Build history of the part. All positions in model axes, mm. Face numbers are marked on the shaded views. A direction names the side the tool comes from. Round coordinates to 2 decimals unless told otherwise and drop trailing zeros. Order: outer loops, then holes, each group sorted by start corner. A loop starts at its lowest first (then second) coordinate and runs counter-clockwise, first axis right, second up. Notation, with made-up numbers: M -27.75,34.5 L 18.25,34.5 A20 ccw 18.25,40.5 Z; hole C 80.5,-14.75 d1. An arc over 180 degrees is marked long. Use CSV: the item, a comma, the result in double quotes.
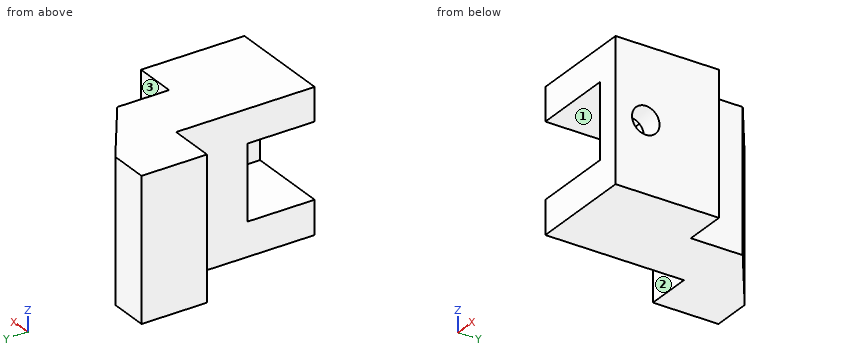
Autodesk Inventor part; units mm, degrees
ref_plane "YZ Plane" through (0, 0, 0) normal (1, 0, 0) x (0, 1, 0)
ref_plane "XZ Plane" through (0, 0, 0) normal (0, 1, 0) x (-1, 0, 0)
ref_plane "XY Plane" through (0, 0, 0) normal (0, 0, 1) x (1, 0, 0)
sketch "草圖1" plane through (0, 0, 0) normal (0, 0, 1) x (1, 0, 0)
  line L0 (20.5635, 0) -> (58.6435, 0)
  line L1 (58.6435, 0) -> (58.6435, 37.62)
  line L2 (58.6435, 37.62) -> (43.3835, 37.62)
  line L3 (43.3835, 37.62) -> (43.3835, 56.4986)
  line L4 (43.3835, 56.4986) -> (17.9968, 74.2368)
  line L5 (17.9968, 74.2368) -> (3.7768, 74.2368)
  line L6 (3.7768, 74.2368) -> (3.7768, 50.4)
  line L7 (3.7768, 50.4) -> (20.5635, 50.4)
  line L8 (20.5635, 50.4) -> (20.5635, 0)
  point P0 (0, 0)
  dimension "d0" = 38.08
  dimension "d1" = 37.62
  dimension "d2" = 15.26
  dimension "d3" = 50.4
  dimension "d4" = 14.22
extrude "擠出1" add sketch "草圖1" along normal blind 51.2
sketch "草圖2" plane through (58.6435, 0, 0) normal (1, 0, 0) x (0, 0, -1)
  circle A0 centre (-25.46, 11) radius 5
  line L0 (0, 37.62) -> (0, 0)
  line L1 (0, 0) -> (-51.2, 0)
  dimension "d7" = 10
  dimension "d8" = 25.46
  dimension "d9" = 11
extrude "擠出2" cut sketch "草圖2" against normal blind 51.2
sketch "草圖3" plane through (20.5635, 0, 0) normal (-1, 0, 0) x (0, 0, 1)
  line L0 (39.2, 0) -> (39.2, 24.4)
  line L1 (39.2, 24.4) -> (12.2, 24.4)
  line L2 (12.2, 24.4) -> (12.2, 0)
  line L3 (51.2, 50.4) -> (51.2, 0)
  line L4 (12.2, 0) -> (12.2, -12.2233)
  line L5 (12.2, -12.2233) -> (39.2, -4.7386)
  line L6 (39.2, -4.7386) -> (39.2, 0)
  dimension "d12" = 27
  dimension "d13" = 12
extrude "擠出3" cut sketch "草圖3" against normal blind 29.64
properties part number "小虎鉗-右側" material "鋁合金 6061"
(1) Wall check: line 1 (Y direction, x = 57, z = 25.46); line 2 (Y direction, x = 44, z = 35); line 3 (Y direction, x = 53, z = 43). Give the ranges that are in metal, low to high. Write a range as from..to.
Answer block:
line 1,"y = 0..6, 16..37.62"
line 2,"y = 24.4..37.62"
line 3,"y = 0..37.62"
(2) Drop flat-ended pins along their axis: pin 1 (8 mm diameter, centred on x = 39.5, z = 29.5, fed in from -Y); pin 2 (12 mm diameter, centred on y = 41.5, z = 21.5, fed in from +X); pin 3 (8 mm diameter, centred on y = 22, z = 12.5, fed in from -X); pin 4 (7.5 mm diameter, centred on x = 53, z = 33, fed in from +Y). Give the stop position or say it passes through.
Answer block:
pin 1,"stops at y = 24.4"
pin 2,"stops at x = 58.64"
pin 3,"stops at x = 20.56"
pin 4,"stops at y = 37.62"
(3) Cut at C-C, the plane y = 11. Give the cut face in (x, z), and give its area (3 significant figures).
Answer block:
outline,"M 20.56,0 L 58.64,0 L 58.64,20.46 L 50.2,20.46 L 50.2,12.2 L 20.56,12.2 Z; M 20.56,39.2 L 50.2,39.2 L 50.2,30.46 L 58.64,30.46 L 58.64,51.2 L 20.56,51.2 Z"
area,"1,070 mm²"
(4) Cut at A-A, the plane y = 20.5. Give the cut face in (x, z), and give its area (3 significant figures).
Answer block:
outline,"M 20.56,0 L 58.64,0 L 58.64,51.2 L 20.56,51.2 L 20.56,39.2 L 50.2,39.2 L 50.2,12.2 L 20.56,12.2 Z"
area,"1,150 mm²"
(5) Cut at B-B, the plane z = 25.46. Give the cut face in (x, y).
Answer block:
outline,"M 3.78,50.4 L 20.56,50.4 L 20.56,24.4 L 50.2,24.4 L 50.2,16 L 58.64,16 L 58.64,37.62 L 43.38,37.62 L 43.38,56.5 L 18,74.24 L 3.78,74.24 Z; M 50.2,0 L 58.64,0 L 58.64,6 L 50.2,6 Z"
(6) Tool access for the marked faces 1, 2 and 3: list every direction of +Z, -Z, +X, -X, +Y, -Y with a clear straight run to the whole face (end or side of a thin tool).
Answer block:
face 1,"-X, -Y"
face 2,"+Z, -Z, -X, -Y"
face 3,"+Z, -Z, +X, +Y"
(7) Cut at D-D, the plane x = 32. Give the cut face in (y, z), and give its area (3 significant figures).
Answer block:
outline,"M 0,0 L 64.45,0 L 64.45,51.2 L 0,51.2 L 0,39.2 L 24.4,39.2 L 24.4,12.2 L 0,12.2 Z"
area,"2,640 mm²"
